For this review, take the finished solid that the model builds, in its own axes (mm). Face numbers are marked on the shaded views. A direction names the side the tool comes from. Coordinates: 2 decimals unless noted, no trailing zeros. Loops run counter-clockwise (first coordinate to the right, second up) from the corner with the lowest first, then second, coordinate; pieces in that order, holes last. Notation, with made-up numbers: (74, 18) - (121, 18) arc R19 ccw to (121, 35) - close; hole circle Ø9 at (1, 46.25). An arc over 180 degrees is marked (long way). Use one line per item in the form item = value. Start each with the question number.
1. Add section A-A on z = 0. Give the boundary of the cut face in (x, y), and give its area (3 significant figures).
2. Draft analysis for pull direction Z (two halves, no side actions). For the marked faces 1, 2 and 3, state which applies: +Z half, -Z half, draft (parallel to the pull), parting line (faces both ways), or undercut.
3. Add section C-C on y = 7. Give the boundary of the cut face in (x, z).
4. To check wall thickness, follow probe 1 along Z at (x, y) = (-109.88, 4.5); probe 2 along X at (y, z) = (3.75, -3); probe 3 along Z at (x, y) = (-104.5, 5). State the ranges of each line that lie inside material, in increasing order.
5. Add section B-B on x = -128. Give the boundary of the cut face in (y, z).
6. For pin 1 Ø5 at (x, y) = (-60, 5) entering from +Z; pin 2 Ø1 at (y, z) = (8, 0) entering from -X; pin 3 Ø4 at (y, z) = (8.5, 38.5) entering from +X, all flat-tipped, find the tip position at first contact; note any pin that passes through.
7. Add section D-D on x = -109.88. Give the boundary of the cut face in (y, z).
8. Machinability: for the marked faces 4 and 5, which of the approach directions +Z, -Z, +X, -X, +Y, -Y give a long, thin tool a straight path to every point of the face, cutting with its end or side? Answer none if there is none.
Autodesk Inventor part; units mm, degrees
ref_plane "YZ Plane" through (0, 0, 0) normal (1, 0, 0) x (0, 1, 0)
ref_plane "XZ Plane" through (0, 0, 0) normal (0, 1, 0) x (-1, 0, 0)
ref_plane "XY Plane" through (0, 0, 0) normal (0, 0, 1) x (1, 0, 0)
sketch "Sketch1" plane through (0, 0, 0) normal (0, 1, 0) x (-1, 0, 0)
  arc A0 (0, 15) -> (0, -15) centre (0, 0) ccw
  line L0 (0, -15) -> (130.51, -15)
  line L1 (0, 15) -> (83, 15)
  arc A1 (130.51, -15) -> (145.1737, -3.1586) centre (130.51, 0) ccw
  arc A2 (123.667, 1.474) -> (137.353, -1.474) centre (130.51, 0) ccw
  circle A3 centre (109.88, 0) radius 7
  arc A4 (123.667, 1.474) -> (104.1154, 25.6855) centre (104.1154, 5.6855) ccw
  arc A5 (104.1154, 39.6855) -> (104.1154, 25.6855) centre (104.1154, 32.6855) ccw
  arc A6 (137.353, -1.474) -> (104.1154, 39.6855) centre (104.1154, 5.6855) ccw
  arc A7 (104.1154, 47.6855) -> (90, 37.7605) centre (104.1154, 32.6855) ccw
  line L2 (90, 22) -> (90, 37.7605)
  arc A8 (145.1737, -3.1586) -> (104.1154, 47.6855) centre (104.1154, 5.6855) ccw
  arc A9 (83, 15) -> (90, 22) centre (83, 22) ccw
  point P0 (90, 15)
  dimension "d0" = 30
  dimension "d1" = 130.51
  dimension "d2" = 90
  dimension "d3" = 15
  dimension "d4" = 14
  dimension "d5" = 20.63
  dimension "d6" = 14
  dimension "d9" = 20
  dimension "d11" = 14
  dimension "d12" = 15
  dimension "d13" = 42
  dimension "d14" = 7
extrude "Extrusion1" add sketch "Sketch1" along normal blind 10
properties part number "Assignment#1"
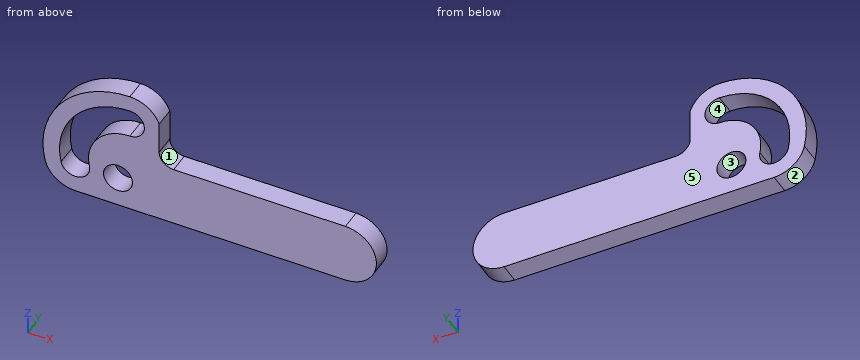
Conclusion:
q1.outline = (-145.73, 0) - (-137.64, 0) - (-137.64, 10) - (-145.73, 10) - close; (-123.51, 0) - (-116.88, 0) - (-116.88, 10) - (-123.51, 10) - close; (-102.88, 0) - (15, 0) - (15, 10) - (-102.88, 10) - close
q1.area = 1,330 mm^2
q2.face_1 = +Z half
q2.face_2 = -Z half
q2.face_3 = undercut
q3.outline = (-145.17, -3.16) arc R15 ccw to (-130.51, -15) - (0, -15) arc R15 ccw to (0, 15) - (-83, 15) arc R7 cw to (-90, 22) - (-90, 37.76) arc R15 ccw to (-104.12, 47.69) arc R42 ccw to start; hole (-137.35, -1.47) arc R7 ccw to (-123.67, 1.47) arc R20 cw to (-104.12, 25.69) arc R7 ccw to (-104.12, 39.69) arc R34 ccw to start; hole circle Ø14 at (-109.88, 0)
q4.probe_1 = -15 to -7, 7 to 24.84, 39.19 to 47.29
q4.probe_2 = -145.21 to -136.83, -124.19 to -116.2, -103.56 to 14.7
q4.probe_3 = -15 to -4.48, 4.48 to 25.68, 39.68 to 47.68
q5.outline = (0, -15) - (10, -15) - (10, -6.53) - (0, -6.53) - close; (0, 29.88) - (10, 29.88) - (10, 40.23) - (0, 40.23) - close
q6.pin_1 = 15
q6.pin_2 = -145.79
q6.pin_3 = -90
q7.outline = (0, -15) - (10, -15) - (10, -7) - (0, -7) - close; (0, 7) - (10, 7) - (10, 24.84) - (0, 24.84) - close; (0, 39.19) - (10, 39.19) - (10, 47.29) - (0, 47.29) - close
q8.face_4 = +Y, -Y
q8.face_5 = +Z, -Z, +X, -X, +Y
